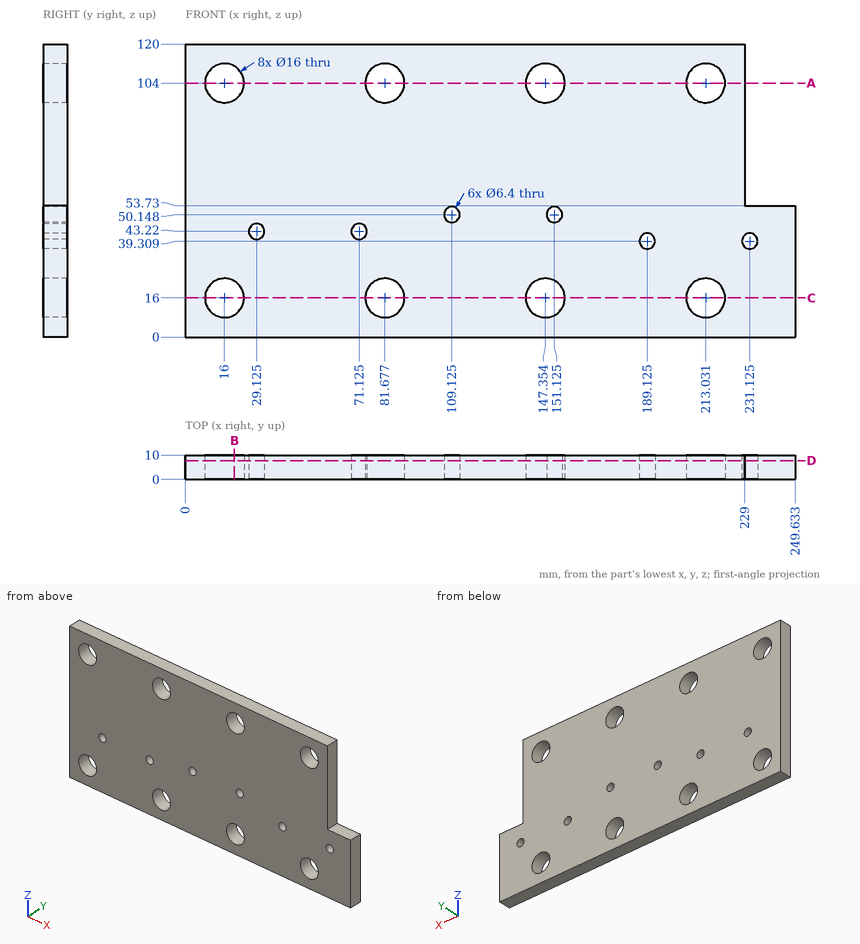
Here's the drawing with two shaded views (mm, measured from the low corner). I have some questions. Round coordinates to 2 decimals unless told otherwise and drop trailing zeros. Loops run counter-clockwise (first coordinate to the right, second up) from the corner with the lowest first, then second, coordinate; pieces in that order, holes last.
Item 1: Suppose I cut it at B-B, the plane x = 20. Write out the boundary of the cut face in (y, z).
Item 2: Suppose I cut it at D-D, the plane y = 7.75. State how many separate pieces and enclosed holes the cut face has, then the cut area to 3 significant figures.
Item 3: Suppose I cut it at A-A, the plane z = 104. Write out the boundary of the cut face in (x, y) (1 decimal).
Item 4: Will this pin go through, and if not, where does the flat tip stop? pin 1 Ø10 at (x, z) = (109.12, 50.15) entering from +Y.
Item 5: Suppose I cut it at C-C, the plane z = 16. Write out the boundary of the cut face in (x, y) (1 decimal).
Item 6: Please list where these lines run through material, in increasing order: L1, parallel to Z at x = 16, y = 7.5; L2, parallel to X at y = 9, z = 107 (1 decimal); L3, parallel to Z at x = 88.5, y = 8.5 (1 decimal).
Reported:
1. outline: (0, 0) - (10, 0) - (10, 9.07) - (0, 9.07) - close; (0, 22.93) - (10, 22.93) - (10, 97.07) - (0, 97.07) - close; (0, 110.93) - (10, 110.93) - (10, 120) - (0, 120) - close
2. separate pieces: 1
2. enclosed holes: 14
2. area: 26,800 mm2
3. outline: (0, 0) - (8, 0) - (8, 10) - (0, 10) - close; (24, 0) - (73.7, 0) - (73.7, 10) - (24, 10) - close; (89.7, 0) - (139.4, 0) - (139.4, 10) - (89.7, 10) - close; (155.4, 0) - (205, 0) - (205, 10) - (155.4, 10) - close; (221, 0) - (229, 0) - (229, 10) - (221, 10) - close
4. pin 1: stops at y = 10
5. outline: (0, 0) - (8, 0) - (8, 10) - (0, 10) - close; (24, 0) - (73.7, 0) - (73.7, 10) - (24, 10) - close; (89.7, 0) - (139.4, 0) - (139.4, 10) - (89.7, 10) - close; (155.4, 0) - (205, 0) - (205, 10) - (155.4, 10) - close; (221, 0) - (249.6, 0) - (249.6, 10) - (221, 10) - close
6. L1: z = 0 to 8, 24 to 96, 112 to 120
6. L2: x = 0 to 8.6, 23.4 to 74.3, 89.1 to 139.9, 154.8 to 205.6, 220.4 to 229
6. L3: z = 0 to 11.8, 20.2 to 99.8, 108.2 to 120
